```python
from build123d import *

# Parameters (mm, degrees)
CROQUIS1_R              = 1.55
CROQUIS1_R_2            = 2.55
CROQUIS1_R_3            = 2.5
CROQUIS1_W              = 3.2
CROQUIS1_H              = 6
SALIENTE_EXTRUIR1_DEPTH = 3
REDONDEO2_R             = 2


with BuildPart() as part:
    # Croquis1 → Saliente-Extruir1 (new body)
    with BuildSketch(Plane(origin=(0, 0, 0), x_dir=(1, 0, 0), z_dir=(0, 1, 0))):
        Polygon((0, 0), (275, 0), (275, 31), (229.5, 31), (229.5, 39), (215.5, 39), (215.5, 31), (59.5, 31), (59.5, 39), (45.5, 39), (45.5, 31), (0, 31), align=None)
        with Locations((5, 15)):
            Circle(CROQUIS1_R, mode=Mode.SUBTRACT)
        with Locations((270, 15)):
            Circle(CROQUIS1_R, mode=Mode.SUBTRACT)
        with Locations((10, 27.1)):
            Circle(CROQUIS1_R_2, mode=Mode.SUBTRACT)
        with Locations((33.2, 27.1)):
            Circle(CROQUIS1_R_2, mode=Mode.SUBTRACT)
        with Locations((33.2, 3.9)):
            Circle(CROQUIS1_R_2, mode=Mode.SUBTRACT)
        with Locations((10, 3.9)):
            Circle(CROQUIS1_R_2, mode=Mode.SUBTRACT)
        with Locations((265, 3.9)):
            Circle(CROQUIS1_R_2, mode=Mode.SUBTRACT)
        with Locations((241.8, 3.9)):
            Circle(CROQUIS1_R_2, mode=Mode.SUBTRACT)
        with Locations((265, 27.1)):
            Circle(CROQUIS1_R_2, mode=Mode.SUBTRACT)
        with Locations((241.8, 27.1)):
            Circle(CROQUIS1_R_2, mode=Mode.SUBTRACT)
        with Locations((139, 25)):
            Circle(CROQUIS1_R, mode=Mode.SUBTRACT)
        with Locations((139, 5)):
            Circle(CROQUIS1_R, mode=Mode.SUBTRACT)
        with Locations((52.5, 22)):
            Circle(CROQUIS1_R, mode=Mode.SUBTRACT)
        with Locations((52.5, 4)):
            Circle(CROQUIS1_R, mode=Mode.SUBTRACT)
        with Locations((222.5, 22)):
            Circle(CROQUIS1_R, mode=Mode.SUBTRACT)
        with Locations((222.5, 4)):
            Circle(CROQUIS1_R, mode=Mode.SUBTRACT)
        with Locations((212.5, 26)):
            Circle(CROQUIS1_R, mode=Mode.SUBTRACT)
        with Locations((62.5, 26)):
            Circle(CROQUIS1_R, mode=Mode.SUBTRACT)
        with Locations((201.5, 26)):
            Circle(CROQUIS1_R, mode=Mode.SUBTRACT)
        with Locations((73.5, 26)):
            Circle(CROQUIS1_R, mode=Mode.SUBTRACT)
        with Locations((207, 18)):
            Circle(CROQUIS1_R_3, mode=Mode.SUBTRACT)
        with Locations((68, 18)):
            Circle(CROQUIS1_R_3, mode=Mode.SUBTRACT)
        with Locations((270, 4.5)):
            Rectangle(CROQUIS1_W, CROQUIS1_H, mode=Mode.SUBTRACT)
        with Locations((5, 25.5)):
            Rectangle(CROQUIS1_W, CROQUIS1_H, mode=Mode.SUBTRACT)
        with Locations((5, 4.5)):
            Rectangle(CROQUIS1_W, CROQUIS1_H, mode=Mode.SUBTRACT)
        with Locations((270, 25.5)):
            Rectangle(CROQUIS1_W, CROQUIS1_H, mode=Mode.SUBTRACT)
    extrude(amount=SALIENTE_EXTRUIR1_DEPTH)

    # Redondeo2
    redondeo2_edges = [part.edges().sort_by_distance(p)[0] for p in [
        (0, 1.5, -31),
        (45.5, 1.5, -31),
        (45.5, 1.5, -39),
        (59.5, 1.5, -39),
        (59.5, 1.5, -31),
        (215.5, 1.5, -31),
        (215.5, 1.5, -39),
        (229.5, 1.5, -39),
        (229.5, 1.5, -31),
        (275, 1.5, -31),
        (275, 1.5, 0),
        (0, 1.5, 0),
    ]]
    fillet(redondeo2_edges, radius=REDONDEO2_R)


solid = part.part
```
Work out the finished part from the listing and answer in its coordinate system (mm). Coordinates: 2 decimals unless noted, no trailing zeros. Loops run counter-clockwise (first coordinate to the right, second up) from the corner with the lowest first, then second, coordinate; pieces in that order, holes last.
1) Section B-B (x = 20) is taken. Give the vertices of the cut face in (y, z).
Results:
outline: (0, -31) - (3, -31) - (3, 0) - (0, 0) - close
2) Flat-ended cylindrical pins translate along their axes: pin 1 (1 mm diameter, centred on x = 167, y = 0.5, fed in from -Z); pin 2 (1.5 mm diameter, centred on y = 2, z = -35, fed in from +X); pin 3 (1.5 mm diameter, centred on y = 2, z = -35, fed in from -X). Find the tip coordinate at first contact, or state that the pin passes through.
Results:
pin 1: stops at z = -31
pin 2: stops at x = 229.5
pin 3: stops at x = 45.5
3) For a pull along X with two mould halves and no side action, classify faces 1 (the cylindrical face through (11.18, 1.48, -24.84)), 2 (the cylindrical face through (69.34, 1.48, -20.11)), 3 (the flat face through (136, 0, -15)) as +X half, -X half, draft (parallel to the pull), parting line (faces both ways), or undercut.
Results:
face 1: undercut
face 2: undercut
face 3: draft
4) Consider probe 1 along Z at (x, y) = (52.5, 1.7); probe 2 along Z at (x, y) = (265, 1.25); probe 3 along X at (y, z) = (1.1, -18). Determine where each line is inside the solid, lowest interval first.
Results:
probe 1: z = -39 to -23.55, -20.45 to -5.55, -2.45 to 0
probe 2: z = -31 to -29.65, -24.55 to -6.45, -1.35 to 0
probe 3: x = 0 to 65.5, 70.5 to 204.5, 209.5 to 275
5) Section A-A (y = 2.45) is taken. Give the number of separate pieces and of enclosed holes in the cut face, plus the area to 3 significant figures.
Results:
separate pieces: 1
enclosed holes: 26
area: 8,380 mm2
